from build123d import *


with BuildPart() as f1:
    # F0 (on Front) → F1 (revolve)
    with BuildSketch(Plane.XZ):
        with BuildLine():
            Line((0, 53.65608), (0, 0))
            Line((0, 0), (100, 0))
            Line((100, 0), (100, 24.115275))
            ThreePointArc((100, 24.115275), (99.748956, 24.777895), (99.121869, 25.107821))
            Line((99.121869, 25.107821), (86.868069, 26.612398))
            ThreePointArc((86.868069, 26.612398), (85.613896, 27.272251), (85.111808, 28.597491))
            Line((85.111808, 28.597491), (85.111808, 38.943315))
            ThreePointArc((85.111808, 38.943315), (84.860763, 39.605935), (84.233677, 39.935861))
            Line((84.233677, 39.935861), (71.979877, 41.440439))
            ThreePointArc((71.979877, 41.440439), (70.725704, 42.100291), (70.223615, 43.425531))
            Line((70.223615, 43.425531), (70.223615, 53.65608))
            Line((70.223615, 53.65608), (0, 53.65608))
        make_face()
    revolve(axis=Axis((35.111808, 0, 53.65608), (-1, 0, 0)))


solid = f1.part
The listing builds one solid part. Answer for the finished solid, in the listing's coordinates (mm). A direction names the side the tool comes from. Round coordinates to 2 decimals unless told otherwise and drop trailing zeros. Loops run counter-clockwise (first coordinate to the right, second up) from the corner with the lowest first, then second, coordinate; pieces in that order, holes last. Notation, with made-up numbers: M -40,-22.75 L 1,-22.75 A14 ccw 1,2.25 Z; hole C -32.75,82 d9. An arc over 180 degrees is marked long. Return JSON: item names as keys, results as strings.
Q1. Find section D-D, the plane z = 19.5. Determine the outline of the cut face in (x, y).
Results list:
{"outline": "M 0,-41.38 L 100,-41.38 L 100,41.38 L 0,41.38 Z"}
Q2. Find section C-C, the plane x = 92. Determine the outline of the cut face in (y, z), plus the area to 3 significant figures.
Results list:
{"outline": "C 0,53.66 d107.31; hole C 0,53.66 d55.35", "area": "6,640 mm2"}
Q3. Which of the six approach directions +Z, -Z, +X, -X, +Y, -Y give full straight-line access (tool end or side, diameter ignored) to faces 1 (the face through (85.112, 11, 43)), 2 (the face through (100, 23, 31))?
Results list:
{"face 1": "+X", "face 2": "+Z, -Z, +X, +Y, -Y"}
Q4. Find the intervals of material crossed by line 1 along X through (y, z) = (-15, 54); line 2 along Z through (x, y) = (89, 24.5); line 3 along X through (y, z) = (3, 51.5), in increasing order. Write a range as from..to.
Results list:
{"line 1": "x = 0..85.11", "line 2": "z = 5.92..41.6, 65.71..101.39", "line 3": "x = 0..70.22"}
Q5. Find section B-B, the plane x = 50. Determine the outline of the cut face in (y, z).
Results list:
{"outline": "C 0,53.66 d107.31"}
Q6. The mould has two halves that part along Y. Classify faces 3 (the face through (50.7, 32.649, 96.236)), 4 (the face through (0, -1, 53)), 5 (the face through (76.66, 4.9, 41.84)): released by +Y, released by -Y, zero draft, split by the parting line, or undercut.
Results list:
{"face 3": "split by the parting line", "face 4": "zero draft", "face 5": "undercut"}
Q7. Find section A-A, the plane y = 0. Determine the outline of the cut face in (x, z), plus the area to 3 significant figures.
Results list:
{"outline": "M 0,0 L 100,0 L 100,24.12 A1 ccw 99.12,25.11 L 86.87,26.61 A2 cw 85.11,28.6 L 85.11,38.94 A1 ccw 84.23,39.94 L 71.98,41.44 A2 cw 70.22,43.43 L 70.22,63.89 A2 cw 71.98,65.87 L 84.23,67.38 A1 ccw 85.11,68.37 L 85.11,78.71 A2 cw 86.87,80.7 L 99.12,82.2 A1 ccw 100,83.2 L 100,107.31 L 0,107.31 Z", "area": "9,520 mm2"}
Q8. Each of these flat-tipped pins is pushed along its axis until it touches: pin 1 Ø1.5 at (x, y) = (78.5, 28.5) entering from +Z; pin 2 Ø5 at (x, z) = (52.5, 41) entering from +Y; pin 3 Ø10 at (y, z) = (-4, 58) entering from +X. Where does it stop, or does it pass through?
Results list:
{"pin 1": "stops at z = 99.58", "pin 2": "stops at y = 52.69", "pin 3": "stops at x = 70.34"}
